For this review, take the finished solid that the model builds, in its own axes (mm). Face numbers are marked on the shaded views. A direction names the side the tool comes from. Round coordinates to 2 decimals unless told otherwise and drop trailing zeros. Order: outer loops, then holes, each group sorted by start corner. A loop starts at its lowest first (then second) coordinate and runs counter-clockwise, first axis right, second up. Notation, with made-up numbers: M 14.5,3 L 46.5,3 A17 ccw 46.5,15 Z; hole C 54,-36 d3. An arc over 180 degrees is marked long. Write item = value, one per line. Start each with the question number.
from build123d import *

# Parameters (mm, degrees)
F0_W     = 110.50678
F0_H     = 56.779732
F3_DEPTH = 7.62
F1_W     = 13.002377
F1_H     = 10.885713
F1_W_2   = 12.095236
F1_H_2   = 10.280952
F1_W_3   = 13.002384
F1_W_4   = 12.7
F4_DEPTH = 25.4


with BuildPart() as f3:
    # F0 (on Top) → F3 (new body)
    with BuildSketch(Plane.XY):
        Rectangle(F0_W, F0_H)
    extrude(amount=F3_DEPTH)

    # F1 (on face) → F4 (join)
    with BuildSketch(Plane.XY):
        with Locations((47.624995, 22.690022)):
            Rectangle(F1_W, F1_H)
        with Locations((47.171425, -22.062356)):
            Rectangle(F1_W_2, F1_H_2)
        with Locations((-47.624999, -22.062356)):
            Rectangle(F1_W_3, F1_H_2)
        with Locations((-47.473807, 22.690022)):
            Rectangle(F1_W_4, F1_H)
    extrude(amount=F4_DEPTH)


solid = f3.part
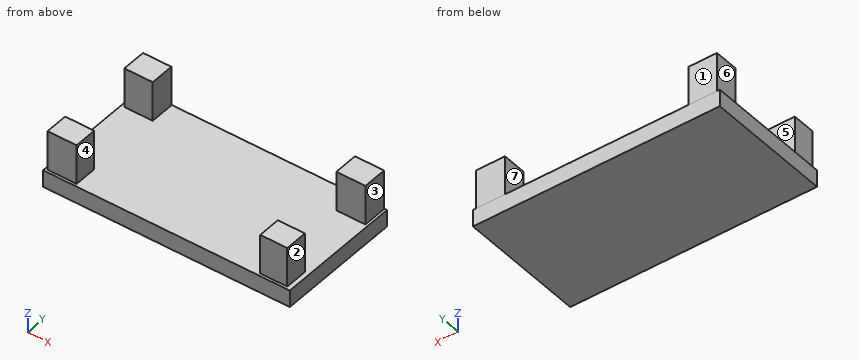
(1) For line 1 along X through (y, z) = (-24.5, 11.5); line 2 along X through (y, z) = (20, 13.25); line 3 along Z through (x, y) = (-13.5, 18.5), list the stretches that pass through material, from the lowest coordinate up.
(2) We need section B-B, the plane x = 46. Write out the cut boundary in (y, z), then the cut area to 3 significant figures.
(3) For the marked faces 1, 2, 3 and 4, list the 3-axis set-ups (+Z, -Z, +X, -X, +Y, -Y) from which the entire face can be reached by the end or side of a thin tool; tool diameter is ignored.
(4) Insertion check: pin 1 (4 mm diameter, centred on y = -15.5, z = 13.5, fed in from -X); pin 2 (13.5 mm diameter, centred on x = 47, z = 13.5, fed in from +Y); pin 3 (4 mm diameter, centred on x = -49, z = 14.5, fed in from +Y); pin 4 (5 mm diameter, centred on x = 26.5, y = 5.5, fed in from +Z). Each pin has a flat end and moves straight along its axis. Give the tip position at first contact, or say it passes through.
(5) Draft analysis for pull direction X (two halves, no side actions). For the marked faces 5, 6 and 7, state which applies: released by +X, released by -X, zero draft, split by the parting line, or undercut.
(6) We need section C-C, the plane y = 21. Write out the cut boundary in (x, z), then the cut area to 3 significant figures.
(7) We need section A-A, the plane z = 9.5. Write out the cut boundary in (x, y).
(8) We need section D-D, the plane x = 3.5. Write out the cut boundary in (y, z), then the cut area to 3 significant figures.
Values:
q1.line_1 = -54.13 to -41.12, 41.12 to 53.22
q1.line_2 = -53.82 to -41.12, 41.12 to 54.13
q1.line_3 = 0 to 7.62
q2.outline = M -28.39,0 L 28.39,0 L 28.39,7.62 L 28.13,7.62 L 28.13,25.4 L 17.25,25.4 L 17.25,7.62 L -16.92,7.62 L -16.92,25.4 L -27.2,25.4 L -27.2,7.62 L -28.39,7.62 Z
q2.area = 809 mm²
q3.face_1 = +Z, +X, -X, +Y
q3.face_2 = +Z, +X, -Y
q3.face_3 = +Z, +X, +Y, -Y
q3.face_4 = +Z, +Y, -Y
q4.pin_1 = -54.13
q4.pin_2 = 28.39
q4.pin_3 = 28.13
q4.pin_4 = 7.62
q5.face_5 = zero draft
q5.face_6 = released by -X
q5.face_7 = undercut
q6.outline = M -55.25,0 L 55.25,0 L 55.25,7.62 L 54.13,7.62 L 54.13,25.4 L 41.12,25.4 L 41.12,7.62 L -41.12,7.62 L -41.12,25.4 L -53.82,25.4 L -53.82,7.62 L -55.25,7.62 Z
q6.area = 1,300 mm²
q7.outline = M -54.13,-27.2 L -41.12,-27.2 L -41.12,-16.92 L -54.13,-16.92 Z; M -53.82,17.25 L -41.12,17.25 L -41.12,28.13 L -53.82,28.13 Z; M 41.12,-27.2 L 53.22,-27.2 L 53.22,-16.92 L 41.12,-16.92 Z; M 41.12,17.25 L 54.13,17.25 L 54.13,28.13 L 41.12,28.13 Z
q8.outline = M -28.39,0 L 28.39,0 L 28.39,7.62 L -28.39,7.62 Z
q8.area = 433 mm²
